For this review, take the finished solid that the model builds, in its own axes (mm). A direction names the side the tool comes from. Give positions to 0.01 mm unless a question says otherwise; leave off trailing zeros. Answer as CSV lines item,"result".
from build123d import *

# Parameters (mm, degrees)
SKETCH_1_R                    = 7.5
SKETCH_1_R_2                  = 5
EXTRUDE_1_DEPTH               = 3
SKETCH_2_W                    = 11
SKETCH_2_H                    = 6
EXTRUDE_2_DEPTH               = 3
SKETCH_5_R                    = 2.5
CUT_EXTRUDE_1_DEPTH           = 1
CUT_EXTRUDE_1_DRAFT           = -37
SKETCH_5_R_2                  = 2.505592327
CUT_EXTRUDE_1_PROFILE_2_DEPTH = 1
CUT_EXTRUDE_1_PROFILE_2_DRAFT = -37
FILLET_2_R                    = 2
SKETCH_7_R                    = 1
CUT_EXTRUDE_3_DEPTH           = 14.647344064
SKETCH_8_W                    = 7.5
SKETCH_8_H                    = 7
EXTRUDE_3_DEPTH               = 3
SKETCH_10_R                   = 2.5
CUT_EXTRUDE_4_DEPTH           = 1
CUT_EXTRUDE_4_DRAFT           = -37
FILLET_3_R                    = 2


with BuildPart() as part:
    # 草图1 → 凸台-拉伸1 (new body)
    with BuildSketch(Plane(origin=(0, 0, 0), x_dir=(0, 0, -1), z_dir=(1, 0, 0))):
        Circle(SKETCH_1_R)
        Circle(SKETCH_1_R_2, mode=Mode.SUBTRACT)
    extrude(amount=EXTRUDE_1_DEPTH)

    # 草图2 → 凸台-拉伸2 (add)
    with BuildSketch(Plane(origin=(3, 0, 0), x_dir=(0, 0, -1), z_dir=(1, 0, 0))):
        with Locations((0, 8)):
            Rectangle(SKETCH_2_W, SKETCH_2_H)
        with Locations((0, -8)):
            Rectangle(SKETCH_2_W, SKETCH_2_H)
    extrude(amount=-EXTRUDE_2_DEPTH)

    # 草图3 → 切除-旋转1 (revolve, cut)
    with BuildSketch(Plane.ZY):
        with BuildLine():
            Line((-2.65, 8), (2.65, 8))
            ThreePointArc((2.65, 8), (0, 5.35), (-2.65, 8))
        make_face()
    revolve(axis=Axis((0, 8, -2.65), (0, 0, 1)), mode=Mode.SUBTRACT)

    # 草图4 → 切除-旋转2 (revolve, cut)
    with BuildSketch(Plane.ZY):
        with BuildLine():
            Line((2.65, -8), (-2.65, -8))
            ThreePointArc((-2.65, -8), (0, -10.65), (2.65, -8))
        make_face()
    revolve(axis=Axis((0, -8, 2.65), (0, 0, -1)), mode=Mode.SUBTRACT)


with BuildPart() as cut_extrude_1_tool:
    # 草图5 → 切除-拉伸1 (with draft: the straight prism first)
    with BuildSketch(Plane(origin=(3, 0, 0), x_dir=(0, 0, -1), z_dir=(1, 0, 0))):
        with Locations((0, 8)):
            Circle(SKETCH_5_R)
    extrude(amount=-CUT_EXTRUDE_1_DEPTH)
    # 切除-拉伸1: the draft: its side faces are tilted about the plane it starts from
    cut_extrude_1_sides = [cut_extrude_1_tool.faces().sort_by_distance(p)[0] for p in [
        (2.5, 8, 2.5),
    ]]
    draft(cut_extrude_1_sides, Plane(origin=(3, 0, 0), x_dir=(0, 0, -1), z_dir=(1, 0, 0)), CUT_EXTRUDE_1_DRAFT)


with BuildPart() as part_1:
    add(part.part)

    # 切除-拉伸1: cut by cut_extrude_1_tool
    add(cut_extrude_1_tool.part, mode=Mode.SUBTRACT)


with BuildPart() as cut_extrude_1_profile_2_tool:
    # 草图5 → 切除-拉伸1 profile 2 (with draft: the straight prism first)
    with BuildSketch(Plane(origin=(3, 0, 0), x_dir=(0, 0, -1), z_dir=(1, 0, 0))):
        with Locations((0, -8)):
            Circle(SKETCH_5_R_2)
    extrude(amount=-CUT_EXTRUDE_1_PROFILE_2_DEPTH)
    # 切除-拉伸1 profile 2: the draft: its side faces are tilted about the plane it starts from
    cut_extrude_1_profile_2_sides = [cut_extrude_1_profile_2_tool.faces().sort_by_distance(p)[0] for p in [
        (2.5, -8, 2.505592327),
    ]]
    draft(cut_extrude_1_profile_2_sides, Plane(origin=(3, 0, 0), x_dir=(0, 0, -1), z_dir=(1, 0, 0)), CUT_EXTRUDE_1_PROFILE_2_DRAFT)


with BuildPart() as part_2:
    add(part_1.part)

    # 切除-拉伸1 profile 2: cut by cut_extrude_1_profile_2_tool
    add(cut_extrude_1_profile_2_tool.part, mode=Mode.SUBTRACT)

    # 圆角2
    fillet_2_edges = [part_2.edges().sort_by_distance(p)[0] for p in [
        (1.5, 11, -5.5),
        (1.5, 11, 5.5),
        (1.5, -11, 5.5),
        (1.5, -11, -5.5),
    ]]
    fillet(fillet_2_edges, radius=FILLET_2_R)

    # 草图7 → 切除-拉伸3 (cut, through all)
    with BuildSketch(Plane(origin=(3, 0, 0), x_dir=(0, 0, -1), z_dir=(1, 0, 0))):
        with Locations((-3.7, -8.5)):
            Circle(SKETCH_7_R)
        with Locations(Location((3.7, -8.5, 0), (0, 0, 180))):
            Circle(SKETCH_7_R)
        with Locations((3.7, 8.5)):
            Circle(SKETCH_7_R)
        with Locations(Location((-3.7, 8.5, 0), (0, 0, 180))):
            Circle(SKETCH_7_R)
    extrude(amount=-CUT_EXTRUDE_3_DEPTH, mode=Mode.SUBTRACT)

    # 草图8 → 凸台-拉伸3 (add)
    with BuildSketch(Plane.ZY):
        with Locations((-9.25, 0)):
            Rectangle(SKETCH_8_W, SKETCH_8_H)
    extrude(amount=-EXTRUDE_3_DEPTH)

    # 草图9 → 切除-旋转3 (revolve, cut)
    with BuildSketch(Plane.ZY):
        with BuildLine():
            Line((-7.35, 0), (-12.65, 0))
            ThreePointArc((-12.65, 0), (-10, 2.65), (-7.35, 0))
        make_face()
    revolve(axis=Axis((0, 0, -7.35), (0, 0, -1)), mode=Mode.SUBTRACT)


with BuildPart() as cut_extrude_4_tool:
    # 草图10 → 切除-拉伸4 (with draft: the straight prism first)
    with BuildSketch(Plane(origin=(3, 0, 0), x_dir=(0, 0, -1), z_dir=(1, 0, 0))):
        with Locations((10, 0)):
            Circle(SKETCH_10_R)
    extrude(amount=-CUT_EXTRUDE_4_DEPTH)
    # 切除-拉伸4: the draft: its side faces are tilted about the plane it starts from
    cut_extrude_4_sides = [cut_extrude_4_tool.faces().sort_by_distance(p)[0] for p in [
        (2.5, 0, -7.5),
    ]]
    draft(cut_extrude_4_sides, Plane(origin=(3, 0, 0), x_dir=(0, 0, -1), z_dir=(1, 0, 0)), CUT_EXTRUDE_4_DRAFT)


with BuildPart() as part_3:
    add(part_2.part)

    # 切除-拉伸4: cut by cut_extrude_4_tool
    add(cut_extrude_4_tool.part, mode=Mode.SUBTRACT)

    # 圆角3
    fillet_3_edges = [part_3.edges().sort_by_distance(p)[0] for p in [
        (1.5, 3.5, -13),
        (1.5, -3.5, -13),
    ]]
    fillet(fillet_3_edges, radius=FILLET_3_R)


solid = part_3.part
1) Wall thickness on line 1 (Y direction, x = 1.2, z = -3.7); line 2 (Z direction, x = 0.5, y = -1); line 3 (Y direction, x = 2, z = 4.5): over which ranges is each line inside the solid? List them lowest first. Write a range as from..to.
From the geometry:
line 1,"y = -10.99..-9.5, -7.5..-3.36, 3.36..7.5, 9.5..10.99"
line 2,"z = -13..-12.4, -7.6..-4.9, 4.9..7.43"
line 3,"y = -10.73..-9.1, -7.9..-2.18, 2.18..7.9, 9.1..10.73"
2) Consider section A-A on x = 1.35. Count the separate pieces of the cut face and the enclosed holes in it, and give its area (3 significant figures).
From the geometry:
separate pieces,"1"
enclosed holes,"8"
area,"165 mm^2"
3) Machinability: for faces 5 (the flat face through (2, 7, 5.5)), 6 (the flat face through (2, -7, -5.5)), 7 (the cylindrical face through (1.48, -10.43, 4.9)), 8 (the flat face through (2, 7, -5.5)), which of the approach directions +Z, -Z, +X, -X, +Y, -Y give a long, thin tool a straight path to every point of the face, cutting with its end or side? Answer none if there is none.
From the geometry:
face 5,"+Z, +X, -X, +Y"
face 6,"-Z, +X, -X, -Y"
face 7,"+Z, +X, -X, -Y"
face 8,"-Z, +X, -X, +Y"
4) Draft analysis for pull direction Z (two halves, no side actions). For faces 1 (the cylindrical face through (1.479, 4.325, -6.127)), 2 (the cylindrical face through (1.52, -9.49, -3.83)), 3 (the flat face through (2, 11, 0)), 4 (the cylindrical face through (1.52, -7.51, 3.83)), state which applies: pulls with the +Z half, pulls with the -Z half, needs draft (parallel to the pull), parting line crosses it, or undercut.
From the geometry:
face 1,"pulls with the -Z half"
face 2,"undercut"
face 3,"needs draft"
face 4,"undercut"
5) Insertion check: P1, Ø1.5, axis at x = 1.5, y = -6.5, coming from the -Z side; P2, Ø1.5, axis at x = 1.5, y = -6, coming from the +Z side. Each pin has a flat end and moves straight along its axis. Give the tip position at first contact, or say it passes through.
From the geometry:
P1,"stops at z = -5.5"
P2,"stops at z = 5.5"
